The model under review builds one solid part; all positions refer to its coordinate system, in mm. Coordinates: 2 decimals unless noted, no trailing zeros. Write each loop counter-clockwise with the first axis right and the second up, starting at its lowest first coordinate (ties: lowest second). Pieces come first, ordered by that corner, then holes.
1) Add section C-C, the plane x = 12. State the section outline as (y, z) points.
2) Add section A-A, the plane y = 40.5. State the section outline as (x, z) points, then the cut area to 3 significant figures.
3) Add section D-D, the plane y = -23. State the section outline as (x, z) points, then the cut area to 3 significant figures.
4) For line 1 (Y direction, x = 1, z = 28); line 2 (Y direction, x = 10.5, z = 24); line 3 (X direction, y = 92.5, z = 37), list the stretches that pass through material, from the lowest coordinate up.
5) Add section B-B, the plane z = 29.5. State the section outline as (x, y) points, then the cut area to 3 significant figures.
from build123d import *

# Parameters (mm, degrees)
F0_W     = 152.4
F0_H     = 266.7
F1_DEPTH = 50.8
F2_R     = 6.35


with BuildPart() as f1:
    # F0 (on Top) → F1 (new body)
    with BuildSketch(Plane.XY):
        with Locations((3.951112, 43.879506)):
            Rectangle(F0_W, F0_H)
        with BuildLine():
            ThreePointArc((23.245994, -26.343299), (-8.652188, -40.408388), (2.476784, -7.371035))
            ThreePointArc((2.476784, -7.371035), (17.044175, -12.27821), (23.245994, -26.343299))
        make_face(mode=Mode.SUBTRACT)
        with BuildLine():
            ThreePointArc((3.522208, 56.067), (17.268992, 50.643009), (23.001112, 37.021828))
            ThreePointArc((23.001112, 37.021828), (16.889747, 23.039903), (2.476784, 18.028965))
            ThreePointArc((2.476784, 18.028965), (-15.091698, 37.545195), (3.522208, 56.067))
        make_face(mode=Mode.SUBTRACT)
        with BuildLine():
            ThreePointArc((24.034084, 100.460825), (17.927302, 86.483142), (3.522208, 81.467))
            ThreePointArc((3.522208, 81.467), (-7.959133, 114.438508), (24.034084, 100.460825))
        make_face(mode=Mode.SUBTRACT)
    extrude(amount=F1_DEPTH)

    # F2
    f2_edges = [f1.edges().sort_by_distance(p)[0] for p in [
        (3.951112, -89.470494, 50.8),
        (80.151112, 43.879506, 50.8),
        (3.951112, 177.229506, 50.8),
        (-72.248888, 43.879506, 50.8),
    ]]
    fillet(f2_edges, radius=F2_R)


solid = f1.part
Geometry results:
1. outline: (-89.47, 0) - (-43.72, 0) - (-43.72, 50.8) - (-83.12, 50.8) arc R6.35 ccw to (-89.47, 44.45) - close; (-8.97, 0) - (19.76, 0) - (19.76, 50.8) - (-8.97, 50.8) - close; (54.29, 0) - (82.75, 0) - (82.75, 50.8) - (54.29, 50.8) - close; (118.17, 0) - (177.23, 0) - (177.23, 44.45) arc R6.35 ccw to (170.88, 50.8) - (118.17, 50.8) - close
2. outline: (-72.25, 0) - (-14.78, 0) - (-14.78, 50.8) - (-65.9, 50.8) arc R6.35 ccw to (-72.25, 44.45) - close; (22.68, 0) - (80.15, 0) - (80.15, 44.45) arc R6.35 ccw to (73.8, 50.8) - (22.68, 50.8) - close
2. area: 5,820 mm2
3. outline: (-72.25, 0) - (-14.56, 0) - (-14.56, 50.8) - (-65.9, 50.8) arc R6.35 ccw to (-72.25, 44.45) - close; (22.95, 0) - (80.15, 0) - (80.15, 44.45) arc R6.35 ccw to (73.8, 50.8) - (22.95, 50.8) - close
3. area: 5,820 mm2
4. line 1: y = -89.47 to -45.12, -7.56 to 18.2, 55.84 to 81.83, 119.09 to 177.23
4. line 2: y = -89.47 to -44.32, -8.37 to 19.13, 54.91 to 82.23, 118.69 to 177.23
4. line 3: x = -72.25 to -12.32, 22.29 to 80.15
5. outline: (-72.25, -89.47) - (80.15, -89.47) - (80.15, 177.23) - (-72.25, 177.23) - close; hole circle Ø38.1 at (4.2, -26.34); hole (3.52, 56.07) arc R19.05 ccw (long way) to (23, 37.02) arc R19.05 ccw to start; hole (3.52, 81.47) arc R19.05 ccw to (24.03, 100.46) arc R19.05 ccw (long way) to start
5. area: 37,200 mm2
